Here's how the part is built. I have some questions about the finished solid (model axes, mm). A direction names the side the tool comes from. Round coordinates to 2 decimals unless told otherwise and drop trailing zeros. Loops run counter-clockwise (first coordinate to the right, second up) from the corner with the lowest first, then second, coordinate; pieces in that order, holes last. Notation, with made-up numbers: M 27.5,-4 L 61.5,-4 A27 ccw 61.5,30 Z; hole C 78,25.5 d7. An arc over 180 degrees is marked long. Write each question's results on one line, items separated by ' | '. Start each with the question number.
```python
from build123d import *

# Parameters (mm, degrees)
F0_W     = 4
F0_H     = 6
F0_H_2   = 12
F0_W_2   = 52
F1_DEPTH = 5


with BuildPart() as f1:
    # F0 (on Top) → F1 (new body)
    with BuildSketch(Plane.XY):
        with Locations((28, 0)):
            Rectangle(F0_W, F0_H)
        with Locations((28, 9)):
            Rectangle(F0_W, F0_H_2)
        Rectangle(F0_W_2, F0_H)
        with Locations((28, -9)):
            Rectangle(F0_W, F0_H_2)
        with Locations((-28, 0)):
            Rectangle(F0_W, F0_H)
        with Locations((-28, 9)):
            Rectangle(F0_W, F0_H_2)
        with Locations((-28, -9)):
            Rectangle(F0_W, F0_H_2)
    extrude(amount=F1_DEPTH)


solid = f1.part
```
Item 1: If we section it at B-B on z = 3.35: Please give me the cut outline in (x, y).
Item 2: Which directions (+Z, -Z, +X, -X, +Y, -Y) give clear straight access to the entire face, cutting with the end or side of a thin tool? Please do faces 5 (the face through (-26, 9, 2)), 6 (the face through (28, -15, 2)), 7 (the face through (0, -3, 2)).
Item 3: I need wall thicknesses on L1, parallel to X at y = -8.25, z = 0.5; L2, parallel to Y at x = 23, z = 1.3. Which ranges of each line are inside material? Lowest first, please.
Item 4: If we section it at C-C on x = 8.5: Please give me the cut outline in (y, z).
Item 5: If we section it at A-A on y = 5.5: Please give me the cut outline in (x, z).
Item 6: If we mould it in two halves opening along X, with no side actions, what happens to faces 1 (the face through (30, 0, 2)), 2 (the face through (26, -9, 2)), 3 (the face through (28, 15, 2)), 4 (the face through (0, 3, 2))? For each: released by +X, released by -X, zero draft, split by the parting line, or undercut.
Numbers:
1) outline: M -30,-15 L -26,-15 L -26,-3 L 26,-3 L 26,-15 L 30,-15 L 30,15 L 26,15 L 26,3 L -26,3 L -26,15 L -30,15 Z
2) face 5: +Z, -Z, +Y | face 6: +Z, -Z, +X, -X, -Y | face 7: +Z, -Z, -Y
3) L1: -30 to -26, 26 to 30 | L2: -3 to 3
4) outline: M -3,0 L 3,0 L 3,5 L -3,5 Z
5) outline: M -30,0 L -26,0 L -26,5 L -30,5 Z; M 26,0 L 30,0 L 30,5 L 26,5 Z
6) face 1: released by +X | face 2: undercut | face 3: zero draft | face 4: undercut
